from build123d import *

# Parameters (mm, degrees)
F1_DEPTH = 62.23
F3_R     = 6.35
F4_DEPTH = 82.551


with BuildPart() as f1:
    # F0 (on Front) → F1 (new body, symmetric)
    with BuildSketch(Plane.XZ):
        Polygon((0, 82.55), (0, 0), (152.4, 0), (133.35, 82.55), align=None)
    extrude(amount=F1_DEPTH, both=True)

    # F2: F1 across plane


with BuildPart() as f1_1:
    add(f1.part)
    add(f1.part.mirror(Plane.YZ))

    # F3 (on face) → F4 (cut, through all)
    with BuildSketch(Plane(origin=(0, 0, 0), x_dir=(1, 0, 0), z_dir=(0, 0, -1))):
        with Locations((127, 0)):
            Circle(F3_R)
        with Locations((-127, 0)):
            Circle(F3_R)
    extrude(amount=-F4_DEPTH, mode=Mode.SUBTRACT)


solid = f1_1.part
Part model, mm, in its own coordinate system. Round coordinates to 2 decimals unless told otherwise and drop trailing zeros. Write each loop counter-clockwise with the first axis right and the second up, starting at its lowest first coordinate (ties: lowest second). Pieces come first, ordered by that corner, then holes. Notation, with made-up numbers: (45, -2.75) - (86, -2.75) arc R28 cw to (86, 18.25) - close; hole circle Ø1 at (51, 84.5). An arc over 180 degrees is marked (long way). Use CSV: the item, a comma, the result in double quotes.
Item 1: Flat gauge pins, fed straight in: P1, Ø4, axis at y = -15, z = 43.5, coming from the +X side; P2, Ø12, axis at y = 44.5, z = 64, coming from the +X side. Where does each tip first touch, or does it go through?
Results list:
P1,"stops at x = 142.82"
P2,"stops at x = 139.02"
Item 2: Pull direction X, two halves, no side cores. Call faces 1 (the flat face through (143.008, -0.871, 40.697)), 2 (the flat face through (2, -62.23, 42)), 3 (the cylindrical face through (-120.943, -1.907, 40.697)): pulls with the +X half, pulls with the -X half, needs draft (parallel to the pull), parting line crosses it, or undercut.
Results list:
face 1,"pulls with the +X half"
face 2,"needs draft"
face 3,"undercut"
Item 3: Slice it at B-B, the plane z = 52. Write the cut outline in (x, y).
Results list:
outline,"(-140.4, -62.23) - (140.4, -62.23) - (140.4, 62.23) - (-140.4, 62.23) - close; hole circle Ø12.7 at (-127, 0); hole circle Ø12.7 at (127, 0)"
Item 4: Wall check: L1, parallel to X at y = 3.5, z = 6.5; L2, parallel to X at y = 0, z = 17; L3, parallel to Y at x = 127, z = 26.5. Give the ranges that are in metal, low to high.
Results list:
L1,"x = -150.9 to -132.3, -121.7 to 121.7, 132.3 to 150.9"
L2,"x = -148.48 to -133.35, -120.65 to 120.65, 133.35 to 148.48"
L3,"y = -62.23 to -6.35, 6.35 to 62.23"
Item 5: Slice it at C-C, the plane y = 14.5. Write the cut outline in (x, z).
Results list:
outline,"(-152.4, 0) - (152.4, 0) - (133.35, 82.55) - (-133.35, 82.55) - close"
Item 6: Slice it at A-A, the plane x = 127. Write the cut outline in (y, z).
Results list:
outline,"(-62.23, 0) - (-6.35, 0) - (-6.35, 82.55) - (-62.23, 82.55) - close; (6.35, 0) - (62.23, 0) - (62.23, 82.55) - (6.35, 82.55) - close"
Item 7: Slice it at D-D, the plane z = 10.5. Write the cut outline in (x, y), then the cut area to 3 significant figures.
Results list:
outline,"(-149.98, -62.23) - (149.98, -62.23) - (149.98, 62.23) - (-149.98, 62.23) - close; hole circle Ø12.7 at (-127, 0); hole circle Ø12.7 at (127, 0)"
area,"37,100 mm²"
